The model under review builds one solid part; all positions refer to its coordinate system, in mm. A direction names the side the tool comes from. Round coordinates to 2 decimals unless told otherwise and drop trailing zeros. Write each loop counter-clockwise with the first axis right and the second up, starting at its lowest first coordinate (ties: lowest second). Pieces come first, ordered by that corner, then holes. Notation, with made-up numbers: (63, -9.75) - (92, -9.75) arc R28 cw to (92, 17.25) - close; hole circle Ø5 at (-36.75, 37.25). An arc over 180 degrees is marked (long way). Write each question's results on one line, items separated by ' | '.
Autodesk Inventor part; units mm, degrees
ref_plane "YZ Plane" through (0, 0, 0) normal (1, 0, 0) x (0, 1, 0)
ref_plane "XZ Plane" through (0, 0, 0) normal (0, 1, 0) x (-1, 0, 0)
ref_plane "XY Plane" through (0, 0, 0) normal (0, 0, 1) x (1, 0, 0)
sketch "Sketch1" plane through (0, 0, 0) normal (0, 1, 0) x (-1, 0, 0)
  line L0 (-10, -60) -> (-50, -60)
  line L1 (-60, -50) -> (-60, -10)
  line L2 (-50, 0) -> (-10, 0)
  line L3 (0, -10) -> (0, -50)
  arc A0 (-60, -50) -> (-50, -60) centre (-50, -50) ccw
  arc A1 (-10, -60) -> (0, -50) centre (-10, -50) ccw
  arc A2 (0, -10) -> (-10, 0) centre (-10, -10) ccw
  arc A3 (-50, 0) -> (-60, -10) centre (-50, -10) ccw
  circle A4 centre (-10, -50) radius 3
  circle A5 centre (-50, -50) radius 3
  circle A6 centre (-10, -10) radius 3
  circle A7 centre (-50, -10) radius 3
  point P0 (0, 0)
  point P1 (0, 0)
  point P2 (-30, 0)
  dimension "d0" = 60
  dimension "d1" = 60
  dimension "d2" = 10
  dimension "d3" = 6
extrude "Extrusion1" add sketch "Sketch1" along normal blind 10
sketch "Sketch2" plane through (0, 10, 0) normal (0, 1, 0) x (1, 0, 0)
  line L0 (0, 50) -> (0, 10)
  line L1 (0, 30) -> (60, 30)
  line L2 (60, 10) -> (60, 50)
  line L3 (30, 60) -> (30, 0)
  line L4 (10, 0) -> (50, 0)
  line L5 (50, 60) -> (10, 60)
  circle A0 centre (30, 30) radius 20
  point P0 (0, 0)
  point P1 (30, 0)
  dimension "d6" = 40
extrude "Extrusion2" add sketch "Sketch2" along normal blind 25
chamfer "Chamfer1" distance 5 angle 45 1 edges at (10, 35, -30)
sketch "Sketch3" plane through (0, 0, 0) normal (0, -1, 0) x (1, 0, 0)
  circle A0 centre (30, -30) radius 15
  point P0 (0, 0)
extrude "Extrusion3" cut sketch "Sketch3" against normal blind 20
sketch "Sketch4" plane through (0, 0, 0) normal (0, -1, 0) x (1, 0, 0)
  circle A0 centre (30, -30) radius 20
  point P0 (0, 0)
extrude "Extrusion4" cut sketch "Sketch4" against normal blind 5
sketch "Sketch5" plane through (30, 35, -30) normal (0, 1, 0) x (1, 0, 0)
  circle A0 centre (0, 0) radius 6
  circle A1 centre (0, 0) radius 15
  point P0 (-30, -30)
  dimension "d16" = 12
hole "Hole1" at (30, 35, -30) direction (0, -1, 0) diameter 10.106 end through all
properties part number "Valve Bonnet"
Q1. For probe 1 along Z at (x, y) = (50, 6); probe 2 along Z at (x, y) = (30, 2); probe 3 along Y at (x, z) = (28, -51.5), list the stretches that pass through material, from the lowest coordinate up.
Evaluation:
probe 1: z = -60 to -53, -47 to -13, -7 to 0 | probe 2: z = -60 to -50, -10 to 0 | probe 3: y = 0 to 10
Q2. We need section D-D (y = 25.5). State the section outline as (x, z) points.
Evaluation:
outline: circle Ø40 at (30, -30); hole circle Ø10.11 at (30, -30)
Q3. Tool access review of faces 5 (the cylindrical face through (52.21, 4.93, -52.03)), 6 (the flat face through (36, 20, -30)): name each direction out of +Z, -Z, +X, -X, +Y, -Y from which nothing blocks a thin tool from reaching the whole face with its end or side.
Evaluation:
face 5: +Y, -Y | face 6: -Y
Q4. The part is to be moulded in two halves that separate along Z. For faces 1 (the cylindrical face through (10, 5, -53)), 2 (the flat face through (60, 5, -30)), 3 (the cylindrical face through (49.076, 19.86, -23.993)), 4 (the cylindrical face through (28.48, 27.4, -25.18)), say which applies: released by +Z, released by -Z, zero draft, split by the parting line, or undercut.
Evaluation:
face 1: undercut | face 2: zero draft | face 3: split by the parting line | face 4: undercut
Q5. We need section C-C (z = -52). State the section outline as (x, y) points, plus the area to 3 significant figures.
Evaluation:
outline: (0.2, 0) - (7.76, 0) - (7.76, 10) - (0.2, 10) - close; (12.24, 0) - (47.76, 0) - (47.76, 10) - (12.24, 10) - close; (52.24, 0) - (59.8, 0) - (59.8, 10) - (52.24, 10) - close | area: 507 mm^2
Q6. Insertion check: P1, Ø3, axis at y = 23, z = -21, coming from the +X side; P2, Ø13, axis at x = 30, z = -30, coming from the +Y side; P3, Ø7, axis at x = 10, z = -50, coming from the +Y side; P4, Ø9, axis at x = 22.5, z = -32, coming from the -Y side. Each pin has a flat end and moves straight along its axis. Give the tip position at first contact, or say it passes through.
Evaluation:
P1: stops at x = 48.54 | P2: stops at y = 35 | P3: stops at y = 10 | P4: stops at y = 20
Q7. We need section B-B (y = 33). State the section outline as (x, z) points, plus the area to 3 significant figures.
Evaluation:
outline: circle Ø34 at (30, -30); hole circle Ø10.11 at (30, -30) | area: 828 mm^2
Q8. We need section A-A (z = -30). State the section outline as (x, y) points.
Evaluation:
outline: (0, 0) - (10, 0) - (10, 5) - (15, 5) - (15, 20) - (24.95, 20) - (24.95, 35) - (15, 35) - (10, 30) - (10, 10) - (0, 10) - close; (35.05, 20) - (45, 20) - (45, 5) - (50, 5) - (50, 0) - (60, 0) - (60, 10) - (50, 10) - (50, 30) - (45, 35) - (35.05, 35) - close
